```python
from build123d import *

# Parameters (mm, degrees)
SKETCH1_W           = 117
SKETCH1_H           = 20
BOSS_EXTRUDE1_DEPTH = 5
SKETCH2_W           = 5
SKETCH2_H           = 20
BOSS_EXTRUDE2_DEPTH = 70
SKETCH3_W           = 10
SKETCH3_H           = 117
BOSS_EXTRUDE3_DEPTH = 5
SKETCH4_W           = 5
SKETCH4_H           = 20
BOSS_EXTRUDE4_DEPTH = 20
SKETCH5_W           = 5
SKETCH5_H           = 20
BOSS_EXTRUDE5_DEPTH = 20
SKETCH6_R           = 2
CUT_EXTRUDE1_DEPTH  = 5


with BuildPart() as part:
    # Sketch1 → Boss-Extrude1 (new body)
    with BuildSketch(Plane(origin=(0, 0, 0), x_dir=(0, 0, -1), z_dir=(1, 0, 0))):
        Rectangle(SKETCH1_W, SKETCH1_H)
    extrude(amount=BOSS_EXTRUDE1_DEPTH)

    # Sketch2 → Boss-Extrude2 (add)
    with BuildSketch(Plane(origin=(5, 0, 0), x_dir=(0, 0, -1), z_dir=(1, 0, 0))):
        with Locations((-56, 0)):
            Rectangle(SKETCH2_W, SKETCH2_H)
        with Locations((56, 0)):
            Rectangle(SKETCH2_W, SKETCH2_H)
    extrude(amount=BOSS_EXTRUDE2_DEPTH)

    # Sketch3 → Boss-Extrude3 (add)
    with BuildSketch(Plane.XZ.offset(10)):
        with Locations((5, 0)):
            Rectangle(SKETCH3_W, SKETCH3_H)
    extrude(amount=BOSS_EXTRUDE3_DEPTH)

    # Sketch4 → Boss-Extrude4 (add)
    with BuildSketch(Plane.XY.offset(58.5)):
        with Locations((72.5, 0)):
            Rectangle(SKETCH4_W, SKETCH4_H)
    extrude(amount=BOSS_EXTRUDE4_DEPTH)

    # Sketch5 → Boss-Extrude5 (add)
    with BuildSketch(Plane(origin=(0, 0, -58.5), x_dir=(-1, 0, 0), z_dir=(0, 0, -1))):
        with Locations((-72.5, 0)):
            Rectangle(SKETCH5_W, SKETCH5_H)
    extrude(amount=BOSS_EXTRUDE5_DEPTH)

    # Sketch6 → Cut-Extrude1 (cut)
    with BuildSketch(Plane.ZY.offset(-70)):
        with Locations((-68.5, 0)):
            Circle(SKETCH6_R)
        with Locations((68.5, 0)):
            Circle(SKETCH6_R)
    extrude(amount=-CUT_EXTRUDE1_DEPTH, mode=Mode.SUBTRACT)


solid = part.part
```
For this review, take the finished solid that the model builds, in its own axes (mm). A direction names the side the tool comes from. Round coordinates to 2 decimals unless told otherwise and drop trailing zeros. Write each loop counter-clockwise with the first axis right and the second up, starting at its lowest first coordinate (ties: lowest second). Pieces come first, ordered by that corner, then holes. Notation, with made-up numbers: (-37, 82) -> (-24, 82) arc R27 ccw to (-24, 103) -> close; hole circle Ø11 at (19.25, 75.25). An arc over 180 degrees is marked (long way). Use one line per item in the form item = value.
Q1. Machinability: for faces 4 (the flat face through (5, 0, 1)), 5 (the flat face through (50, -10, -58)), 6 (the flat face through (70, 0, -66)), 7 (the flat face through (75, 0, 66)), which of the approach directions +Z, -Z, +X, -X, +Y, -Y give a long, thin tool a straight path to every point of the face, cutting with its end or side? Answer none if there is none.
Resolved:
face_4 = +X, +Y
face_5 = +Z, -Z, +X, -Y
face_6 = -Z, -X, +Y, -Y
face_7 = +Z, -Z, +X, +Y, -Y
Q2. Consider section D-D (y = -6.75). State the section outline as (x, z) points.
Resolved:
outline = (0, -58.5) -> (70, -58.5) -> (70, -78.5) -> (75, -78.5) -> (75, -53.5) -> (5, -53.5) -> (5, 53.5) -> (75, 53.5) -> (75, 78.5) -> (70, 78.5) -> (70, 58.5) -> (0, 58.5) -> close
Q3. Clearance check with flat-ended pins moving along their axes: pin 1 Ø6 at (y, z) = (-0.5, 71.5) entering from -X; pin 2 Ø6 at (y, z) = (4, -16) entering from +X; pin 3 Ø3.5 at (y, z) = (0, 68.5) entering from +X; pin 4 Ø8 at (x, y) = (21.5, -10) entering from -Z. State where each tip first meets the part, or that it passes through.
Resolved:
pin_1 = 70
pin_2 = 5
pin_3 = through
pin_4 = -58.5
Q4. Consider section C-C (z = 68.5). State the section outline as (x, y) points.
Resolved:
outline = (70, -10) -> (75, -10) -> (75, -2) -> (70, -2) -> close; (70, 2) -> (75, 2) -> (75, 10) -> (70, 10) -> close
Q5. The part is to be moulded in two halves that separate along Z. For faces 1 (the flat face through (75, 0, -66)), 2 (the flat face through (35, 0, 58.5)), 3 (the cylindrical face through (72.465, 0.601, 70.408)), say which applies: released by +Z, released by -Z, zero draft, split by the parting line, or undercut.
Resolved:
face_1 = zero draft
face_2 = released by +Z
face_3 = undercut
Q6. Consider section B-B (y = 0). State the section outline as (x, z) points, then the cut area to 4 significant figures.
Resolved:
outline = (0, -58.5) -> (70, -58.5) -> (70, -66.5) -> (75, -66.5) -> (75, -53.5) -> (5, -53.5) -> (5, 53.5) -> (75, 53.5) -> (75, 66.5) -> (70, 66.5) -> (70, 58.5) -> (0, 58.5) -> close; (70, -78.5) -> (75, -78.5) -> (75, -70.5) -> (70, -70.5) -> close; (70, 70.5) -> (75, 70.5) -> (75, 78.5) -> (70, 78.5) -> close
area = 1,445 mm²
Q7. To check wall thickness, follow probe 1 along Y at (x, z) = (73.7, -68.5); probe 2 along Z at (x, y) = (70.5, -3.75); probe 3 along Z at (x, y) = (63, -9.5). State the ranges of each line that lie inside material, in increasing order. Write a range as from..to.
Resolved:
probe_1 = -10..-2, 2..10
probe_2 = -78.5..-53.5, 53.5..78.5
probe_3 = -58.5..-53.5, 53.5..58.5
Q8. Consider section A-A (x = 16.5). State the section outline as (y, z) points, then the cut area to 3 significant figures.
Resolved:
outline = (-10, -58.5) -> (10, -58.5) -> (10, -53.5) -> (-10, -53.5) -> close; (-10, 53.5) -> (10, 53.5) -> (10, 58.5) -> (-10, 58.5) -> close
area = 200 mm²
